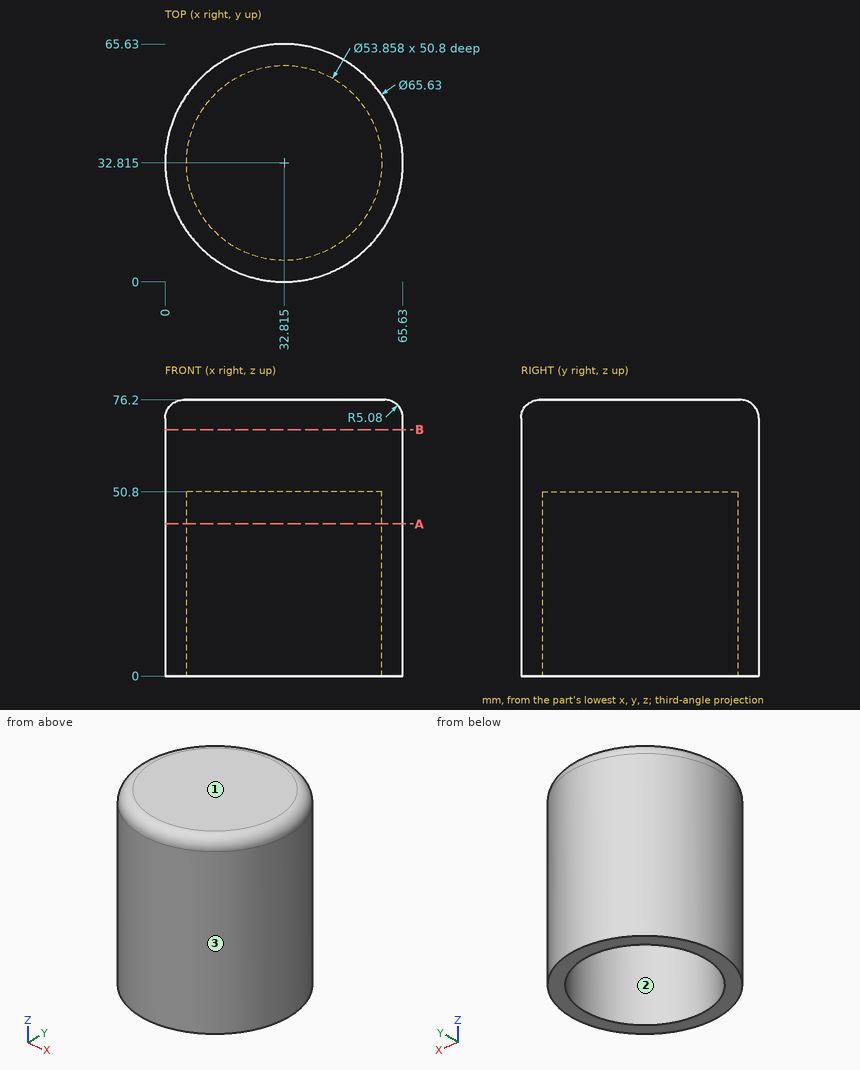
Answer from the drawing. Dimensions are ordinates in mm from the lowest x, y and z of the part. Give positions to 0.01 mm unless a question says otherwise; leave off trailing zeros. Write each loop counter-clockwise with the first axis right and the second up, starting at its lowest first coordinate (ties: lowest second). Pieces come first, ordered by that corner, then holes.
1) Section A-A (z = 42) is taken. Write down the section's boundary in (x, y) (1 decimal).
2) Find the intervals of material crossed by L1, parallel to Z at x = 39, y = 13; L2, parallel to X at y = 32.5, z = 18; L3, parallel to Y at x = 28.5, z = 43 (1 decimal), in increasing order.
3) For a pull along X with two mould halves and no side action, classify the marked faces 1, 2 and 3 as pulls with the +X half, pulls with the -X half, needs draft (parallel to the pull), parting line crosses it, or undercut.
4) Section B-B (z = 68) is taken. Write down the section's boundary in (x, y) (1 decimal).
5) Given P1, Ø12, axis at y = 54, z = 52, coming from the -X side (1 decimal); P2, Ø8, axis at x = 37, z = 20.5, coming from the +Y side; P3, Ø10, axis at y = 30.5, z = 13.5, coming from the +X side; P4, Ø12, axis at x = 52.5, z = 24.5, coming from the -Y side, each flat-ended and moving along its own axis, determine where each tip first touches the part or whether it passes through.
Response:
1. outline: circle Ø65.6 at (32.8, 32.8); hole circle Ø53.9 at (32.8, 32.8)
2. L1: z = 50.8 to 76.2
2. L2: x = 0 to 5.89, 59.74 to 65.63
2. L3: y = 0.3 to 6.2, 59.4 to 65.3
3. face 1: needs draft
3. face 2: undercut
3. face 3: parting line crosses it
4. outline: circle Ø65.6 at (32.8, 32.8)
5. P1: stops at x = 3.7
5. P2: stops at y = 65.63
5. P3: stops at x = 65.63
5. P4: stops at y = 2.99
